Here's how the part is built. I have some questions about the finished solid (model axes, mm). Round coordinates to 2 decimals unless told otherwise and drop trailing zeros. Order: outer loops, then holes, each group sorted by start corner. A loop starts at its lowest first (then second) coordinate and runs counter-clockwise, first axis right, second up. Notation, with made-up numbers: (63.5, 19.25) - (73.5, 19.25) arc R27 ccw to (73.5, 46.25) - close; hole circle Ø10 at (27.5, 49). An arc over 180 degrees is marked (long way). One line per item, written item: value.
from build123d import *

# Parameters (mm, degrees)
BOSS_EXTRUDE1_DEPTH = 1.524
SKETCH2_R           = 2.5019
SKETCH2_R_2         = 3.175
CUT_EXTRUDE1_DEPTH  = 2.524


with BuildPart() as part:
    # Sketch1 → Boss-Extrude1 (new body)
    with BuildSketch(Plane(origin=(0, 0, 0), x_dir=(1, 0, 0), z_dir=(0, 1, 0))):
        Polygon((-50.221590033, -9.319139437), (70.606209967, -9.319139437), (70.606209967, 41.480860563), (35.630409967, 41.480860563), (-15.169590033, 41.480860563), (-50.221590033, 41.480860563), align=None)
    extrude(amount=BOSS_EXTRUDE1_DEPTH)

    # Sketch2 → Cut-Extrude1 (cut, through all)
    with BuildSketch(Plane(origin=(0, 1.524, 0), x_dir=(1, 0, 0), z_dir=(0, 1, 0))):
        with Locations((-37.813690033, -2.969139437)):
            Circle(SKETCH2_R)
        with Locations((58.198309967, -2.969139437)):
            Circle(SKETCH2_R)
        with Locations((32.328409967, 35.130860563)):
            Circle(SKETCH2_R_2)
        with Locations((-8.946590033, 35.130860563)):
            Circle(SKETCH2_R_2)
    extrude(amount=-CUT_EXTRUDE1_DEPTH, mode=Mode.SUBTRACT)


solid = part.part
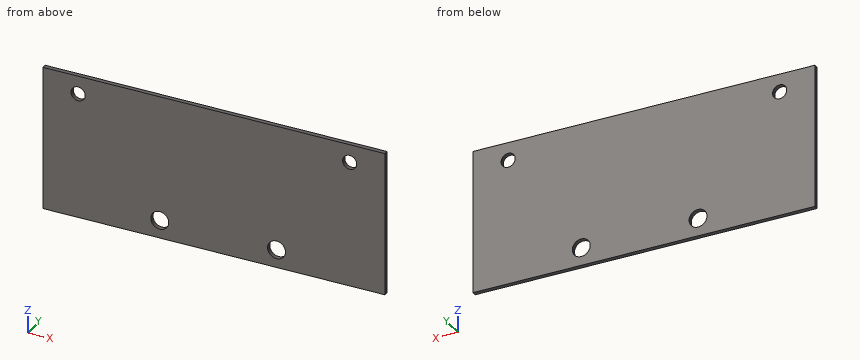
Q1. If I drill on line 1 along X through (y, z) = (0.4, -37.5); line 2 along X through (y, z) = (1.2, 4); line 3 along Z through (x, y) = (32, 0.65), over which ranges is the centre line in solid material (lowest first)?
Results list:
line 1: -50.22 to -11.06, -6.83 to 30.21, 34.44 to 70.61
line 2: -50.22 to -40.09, -35.53 to 55.92, 60.48 to 70.61
line 3: -41.48 to -38.29, -31.97 to 9.32
Q2. If we section it at A-A, the plane z = -36.5: Please give me the cut outline in (x, y), then the cut area to 3 significant figures.
Results list:
outline: (-50.22, 0) - (-11.81, 0) - (-11.81, 1.52) - (-50.22, 1.52) - close; (-6.08, 0) - (29.46, 0) - (29.46, 1.52) - (-6.08, 1.52) - close; (35.19, 0) - (70.61, 0) - (70.61, 1.52) - (35.19, 1.52) - close
area: 167 mm²
Q3. If we section it at B-B, the plane y = 0.85: Please give me the cut outline in (x, z) (3 decimals), then the cut area to 3 significant figures.
Results list:
outline: (-50.222, -41.481) - (70.606, -41.481) - (70.606, 9.319) - (-50.222, 9.319) - close; hole circle Ø5.004 at (-37.814, 2.969); hole circle Ø6.35 at (-8.947, -35.131); hole circle Ø6.35 at (32.328, -35.131); hole circle Ø5.004 at (58.198, 2.969)
area: 6,040 mm²
